from build123d import *

# Parameters (mm, degrees)
SKETCH1_R           = 1.5
BOSS_EXTRUDE1_DEPTH = 1.3
BOSS_EXTRUDE2_START = -1.3
SKETCH2_R           = 1.85
BOSS_EXTRUDE2_DEPTH = 0.8
DOME1_FACE_RADIUS   = 1.5
DOME1_HEIGHT        = 1.2
BOSS_EXTRUDE3_START = -2.1
SKETCH3_W           = 0.5
SKETCH3_H           = 0.3
BOSS_EXTRUDE3_DEPTH = 12
CUT_EXTRUDE1_START  = -14.1
SKETCH4_W           = 0.5
SKETCH4_H           = 0.3
CUT_EXTRUDE1_DEPTH  = 2


with BuildPart() as part:
    # Sketch1 → Boss-Extrude1 (new body, symmetric)
    with BuildSketch(Plane.XY):
        Circle(SKETCH1_R)
    extrude(amount=BOSS_EXTRUDE1_DEPTH, both=True)

    # Sketch2 → Boss-Extrude2 (add)
    with BuildSketch(Plane.XY.offset(BOSS_EXTRUDE2_START)):
        Circle(SKETCH2_R)
    extrude(amount=-BOSS_EXTRUDE2_DEPTH)

    # Dome1: a dome of height H over a round flat face of radius A is a cap of a sphere of radius (A * A + H * H) / (2 * H)
    dome1_r = (DOME1_FACE_RADIUS * DOME1_FACE_RADIUS + DOME1_HEIGHT * DOME1_HEIGHT) / (2 * DOME1_HEIGHT)
    dome1_base = Plane((0, 0, 1.3), z_dir=(0, 0, 1))
    with Locations(dome1_base.offset(DOME1_HEIGHT - dome1_r)):
        dome1_ball = Sphere(dome1_r, mode=Mode.PRIVATE)
    add(split(dome1_ball, bisect_by=dome1_base, keep=Keep.TOP, mode=Mode.PRIVATE))

    # Sketch3 → Boss-Extrude3 (add)
    with BuildSketch(Plane.XY.offset(BOSS_EXTRUDE3_START)):
        with Locations((1.05, 0)):
            Rectangle(SKETCH3_W, SKETCH3_H)
        with Locations((-1.05, 0)):
            Rectangle(SKETCH3_W, SKETCH3_H)
    extrude(amount=-BOSS_EXTRUDE3_DEPTH)

    # Sketch4 → Cut-Extrude1 (cut)
    with BuildSketch(Plane.XY.offset(CUT_EXTRUDE1_START)):
        with Locations((1.05, 0)):
            Rectangle(SKETCH4_W, SKETCH4_H)
    extrude(amount=CUT_EXTRUDE1_DEPTH, mode=Mode.SUBTRACT)


solid = part.part
Here's how the part is built. I have some questions about the finished solid (model axes, mm). A direction names the side the tool comes from. Give positions to 0.01 mm unless a question says otherwise; leave off trailing zeros. Loops run counter-clockwise (first coordinate to the right, second up) from the corner with the lowest first, then second, coordinate; pieces in that order, holes last. Notation, with made-up numbers: (-20, 40) -> (11, 40) arc R24 ccw to (11, 52) -> close; hole circle Ø10 at (-23.5, 33). An arc over 180 degrees is marked (long way). One line per item, written item: value.
Q1. If I drill on line 1 along Z through (x, y) = (0.95, 1.45); line 2 along Y through (x, z) = (0.9, -4); line 3 along Y through (x, z) = (0, 0.25), over which ranges is the centre line in solid material (lowest first)?
Answers follow:
line 1: -2.1 to -1.3
line 2: -0.15 to 0.15
line 3: -1.5 to 1.5
Q2. I'm going to push flat-ended pins straight in: pin 1 Ø1 at (x, y) = (0.5, -1) entering from +Z; pin 2 Ø0.6 at (x, z) = (1, -6) entering from -Y; pin 3 Ø1.5 at (x, z) = (1.5, -7) entering from +Y. Where does each tip first touch, or does it pass through?
Answers follow:
pin 1: z = 2.37
pin 2: y = -0.15
pin 3: y = 0.15
Q3. Suppose I cut it at A-A on z = -9.25. Please give me the cut outline in (x, y).
Answers follow:
outline: (-1.3, -0.15) -> (-0.8, -0.15) -> (-0.8, 0.15) -> (-1.3, 0.15) -> close; (0.8, -0.15) -> (1.3, -0.15) -> (1.3, 0.15) -> (0.8, 0.15) -> close
Q4. On a 3-axis mill with a long thin cutter (end or side, diameter ignored), from which of +Z, -Z, +X, -X, +Y, -Y can I reach the whole of each face in a straight line? I mean faces 1 (the face through (-0.401, -1.806, -1.694)), 2 (the face through (-1.5, 0.07, 0.02)). Say none if no direction works.
Answers follow:
face 1: +Z, -Z
face 2: +Z
Q5. Suppose I cut it at D-D on z = 1. Please give me the cut outline in (x, y).
Answers follow:
outline: circle Ø3 at (0, 0)
